Geometry: final body of the model. Coordinates: model frame, mm. Give positions to 0.01 mm unless a question says otherwise; leave off trailing zeros. Write each loop counter-clockwise with the first axis right and the second up, starting at its lowest first coordinate (ties: lowest second). Pieces come first, ordered by that corner, then holes. Notation, with made-up numbers: (-33, 34) -> (-23, 34) arc R16 ccw to (-23, 59) -> close; hole circle Ø9 at (82, 64). An arc over 180 degrees is marked (long way). Answer as a JSON object with one key per item and string values.
from build123d import *

# Parameters (mm, degrees)
SKETCH1_W              = 609.6
SKETCH1_H              = 609.6
BOSS_EXTRUDE1_DEPTH    = 6.35
CUT_EXTRUDE1_START     = -6.35
CUT_EXTRUDE1_OUTLINE_R = 44.45
CUT_EXTRUDE1_DEPTH     = 6.35


# Read off the part's stored shape, not the designer's step: Cut-Extrude1
with BuildPart() as part:
    # Sketch1 → Boss-Extrude1 (new body)
    with BuildSketch(Plane(origin=(0, 0, 0), x_dir=(1, 0, 0), z_dir=(0, 1, 0))):
        with Locations((-82.357575758, -23.090909091)):
            Rectangle(SKETCH1_W, SKETCH1_H)
    extrude(amount=BOSS_EXTRUDE1_DEPTH)

    # Cut-Extrude1 outline → Cut-Extrude1 (cut)
    with BuildSketch(Plane(origin=(0, 6.35, 0), x_dir=(1, 0, 0), z_dir=(0, 1, 0)).offset(CUT_EXTRUDE1_START)):
        with Locations((-82.357575758, 129.309090909)):
            Circle(CUT_EXTRUDE1_OUTLINE_R)
        with Locations((-82.357575758, 21.359090909)):
            Circle(CUT_EXTRUDE1_OUTLINE_R)
        with Locations((-82.357575758, -111.990909091)):
            Circle(CUT_EXTRUDE1_OUTLINE_R)
        with BuildLine():
            Line((-39.760480786, 281.709090909), (-124.954670729, 281.709090909))
            ThreePointArc((-124.954670729, 281.709090909), (-82.357575758, 249.959090909), (-39.760480786, 281.709090909))
        make_face()
    extrude(amount=CUT_EXTRUDE1_DEPTH, mode=Mode.SUBTRACT)


solid = part.part
Q1. Material intervals for L1, parallel to Z at x = -90, y = 2.5; L2, parallel to Z at x = -113, y = 5.75; L3, parallel to X at y = 1.5, z = -257, sorted ascending. Write a range as from..to.
Values:
{"L1": "-250.62..-173.1, -85.52..-65.15, 22.43..68.2, 155.78..327.89", "L2": "-262.21..-161.51, -97.11..-53.56, 10.84..79.79, 144.19..327.89", "L3": "-387.16..-106.37, -58.35..222.44"}
Q2. Mould query, pull axis Z, two halves, no side actions, for faces 1 (the cylindrical face through (-39.96, 3.13, -142.66)), 2 (the cylindrical face through (-83.155, 3.131, -249.966)), 3 (the flat face through (-154, 0, 19)). Classes: pulls with the +Z half, pulls with the -Z half, needs draft (parallel to the pull), parting line crosses it, or undercut.
Values:
{"face 1": "undercut", "face 2": "pulls with the -Z half", "face 3": "needs draft"}
Q3. Cut plane C-C (x = -95). Return the cut outline in (y, z), and give its area (3 significant figures).
Values:
{"outline": "(0, -251.79) -> (6.35, -251.79) -> (6.35, -171.92) -> (0, -171.92) -> close; (0, -86.69) -> (6.35, -86.69) -> (6.35, -63.97) -> (0, -63.97) -> close; (0, 21.26) -> (6.35, 21.26) -> (6.35, 69.38) -> (0, 69.38) -> close; (0, 154.61) -> (6.35, 154.61) -> (6.35, 327.89) -> (0, 327.89) -> close", "area": "2,060 mm²"}
Q4. Cut plane D-D (z = 93.5). Return the cut outline in (x, y).
Values:
{"outline": "(-387.16, 0) -> (-122.78, 0) -> (-122.78, 6.35) -> (-387.16, 6.35) -> close; (-41.94, 0) -> (222.44, 0) -> (222.44, 6.35) -> (-41.94, 6.35) -> close"}
Q5. Cut plane A-A (z = -6). Return the cut outline in (x, y), and give its area (3 significant figures).
Values:
{"outline": "(-387.16, 0) -> (-124.07, 0) -> (-124.07, 6.35) -> (-387.16, 6.35) -> close; (-40.65, 0) -> (222.44, 0) -> (222.44, 6.35) -> (-40.65, 6.35) -> close", "area": "3,340 mm²"}
Q6. Cut plane B-B (y = 1). Return the cut outline in (x, z), and give its area (3 significant figures).
Values:
{"outline": "(-387.16, -281.71) -> (-124.95, -281.71) arc R44.45 cw to (-39.76, -281.71) -> (222.44, -281.71) -> (222.44, 327.89) -> (-387.16, 327.89) -> close; hole circle Ø88.9 at (-82.36, -129.31); hole circle Ø88.9 at (-82.36, -21.36); hole circle Ø88.9 at (-82.36, 111.99)", "area": "351,000 mm²"}
